```python
from build123d import *

# Parameters (mm, degrees)
F1_DEPTH = 6.35


with BuildPart() as f1:
    # F0 (on Top) → F1 (new body)
    with BuildSketch(Plane.XY):
        with BuildLine():
            Line((-3, 23.152184), (-146.05, 23.152184))
            ThreePointArc((-146.05, 23.152184), (-150.540128, 21.292312), (-152.4, 16.802184))
            Line((-152.4, 16.802184), (-152.4, -53.047816))
            Line((-152.4, -53.047816), (152.4, -53.047816))
            Line((152.4, -53.047816), (152.4, 16.802184))
            ThreePointArc((152.4, 16.802184), (150.540128, 21.292312), (146.05, 23.152184))
            Line((146.05, 23.152184), (3, 23.152184))
            Line((3, 23.152184), (3, -14.947816))
            Line((3, -14.947816), (-3, -14.947816))
            Line((-3, -14.947816), (-3, 23.152184))
        make_face()
    extrude(amount=F1_DEPTH)


solid = f1.part
```
Input: part model. Units: mm. Frame: model coordinates. A direction names the side the tool comes from. Coordinates: 2 decimals unless noted, no trailing zeros. Loops run counter-clockwise (first coordinate to the right, second up) from the corner with the lowest first, then second, coordinate; pieces in that order, holes last. Notation, with made-up numbers: M -6.5,20 L 0.5,20 A22 cw 0.5,40 Z; hole C 16,-5 d8. An arc over 180 degrees is marked long. Use a Markdown table: item, result. Add a question column.
1) Set-up query: faces 1 (the flat face through (152.4, -19, 3)), 2 (the flat face through (0, -14.948, 3)). Return all of +Z, -Z, +X, -X, +Y, -Y with unobstructed straight access to the full face (end or side cutting, diameter ignored); none if empty.
2) Draft query along X for faces 3 (the flat face through (-152.4, -18, 3)), 4 (the flat face through (-2, -53.048, 3)), 5 (the flat face through (3, 4, 3)). Return one class per face: +X half, -X half, draft (parallel to the pull), parting line (faces both ways), or undercut.
3) Line query: L1, parallel to X at y = 15, z = 6; L2, parallel to X at y = 18, z = 5.25. Output: solid intervals per line, ascending. Write a range as from..to.
4) Section A-A, the plane y = 14. Return the cut outline in (x, z), plus the area to 3 significant figures.
Answer below:
| question | item | result |
|---|---|---|
| 1 | face 1 | +Z, -Z, +X, +Y, -Y |
| 1 | face 2 | +Z, -Z, +Y |
| 2 | face 3 | -X half |
| 2 | face 4 | draft |
| 2 | face 5 | undercut |
| 3 | L1 | -152.4..-3, 3..152.4 |
| 3 | L2 | -152.29..-3, 3..152.29 |
| 4 | outline | M -152.4,0 L -3,0 L -3,6.35 L -152.4,6.35 Z; M 3,0 L 152.4,0 L 152.4,6.35 L 3,6.35 Z |
| 4 | area | 1,900 mm2 |
